Autodesk Inventor part; units mm, degrees
ref_plane "YZ Plane" through (0, 0, 0) normal (1, 0, 0) x (0, 1, 0)
ref_plane "XZ Plane" through (0, 0, 0) normal (0, 1, 0) x (-1, 0, 0)
ref_plane "XY Plane" through (0, 0, 0) normal (0, 0, 1) x (1, 0, 0)
sketch "Sketch1" plane through (0, 0, 0) normal (0, 0, 1) x (1, 0, 0)
  line L0 (0, 0) -> (1752.6, 0)
  line L1 (1752.6, 0) -> (1752.6, 304.8)
  line L2 (1752.6, 304.8) -> (0, 304.8)
  line L3 (0, 304.8) -> (0, 0)
  dimension "d0" = 1752.6
  dimension "d1" = 304.8
extrude "Extrusion1" add sketch "Sketch1" against normal blind 6.35
fillet "Fillet1" radius 76.2 2 edges at (0, 304.8, -3.175) (1752.6, 304.8, -3.175)
ref_plane "Work Plane1" through (876.3, 0, 0) normal (1, 0, 0) x (0, 1, 0)
properties part number "FE00036Shelf" material "Aluminum 6061"
CAD build for the part. Positions are in the model's coordinates, mm. Give positions to 0.01 mm unless a question says otherwise; leave off trailing zeros. Loops run counter-clockwise (first coordinate to the right, second up) from the corner with the lowest first, then second, coordinate; pieces in that order, holes last. Notation, with made-up numbers: M 55,62 L 77,62 A23 ccw 77,89 Z; hole C 34.25,5.5 d9. An arc over 180 degrees is marked long. One line per question, with ' | ' between items. Start each with the question number.
1. Probe L1, parallel to X at y = 272.5, z = -5.5; L2, parallel to X at y = 271, z = -3.25. List the from-to ranges inside material, lowest first. Write a range as from..to.
2. Saw through at A-A on y = 274.5. Give the cut face in (x, z), plus the area to 3 significant figures.
3. Flat gauge pin, fed straight in: pin 1 (1.5 mm diameter, centred on x = 1330.5, y = 34, fed in from +Z). Where does the tip first touch, or does it go through?
Result sheet:
1) L1: x = 13.92..1738.68 | L2: x = 12.89..1739.71
2) outline: M 15.38,-6.35 L 1737.22,-6.35 L 1737.22,0 L 15.38,0 Z | area: 10,900 mm^2
3) pin 1: stops at z = 0
